Geometry check sheet. Reference: the model listing, model coordinates, mm. A direction names the side the tool comes from. Coordinates: 2 decimals unless noted, no trailing zeros. Loops run counter-clockwise (first coordinate to the right, second up) from the corner with the lowest first, then second, coordinate; pieces in that order, holes last.
from build123d import *

# Parameters (mm, degrees)
EXTRUSION1_DEPTH = 89
ESQUISSE2_R      = 1.5
ESQUISSE2_W      = 18.5
ESQUISSE2_H      = 20
ESQUISSE2_H_2    = 21.5
EXTRUSION2_DEPTH = 100
ESQUISSE3_R      = 1.5
EXTRUSION3_DEPTH = 100


with BuildPart() as part:
    # Esquisse1 → Extrusion1 (new body)
    with BuildSketch(Plane.XY):
        Polygon((-24.93137059, 6.591473684), (-24.93137059, -13.408526316), (-4.93137059, -13.408526316), (-4.93137059, -11.908526316), (-23.43137059, -11.908526316), (-23.43137059, 6.591473684), align=None)
    extrude(amount=EXTRUSION1_DEPTH)

    # Esquisse2 → Extrusion2 (cut)
    with BuildSketch(Plane(origin=(0, -11.908526316, 0), x_dir=(-1, 0, 0), z_dir=(0, 1, 0))):
        with Locations((14.93137059, 59)):
            Circle(ESQUISSE2_R)
        with Locations((14.93137059, 30)):
            Circle(ESQUISSE2_R)
        with Locations((14.18137059, 79)):
            Rectangle(ESQUISSE2_W, ESQUISSE2_H)
        with Locations((14.18137059, 10.75)):
            Rectangle(ESQUISSE2_W, ESQUISSE2_H_2)
    extrude(amount=-EXTRUSION2_DEPTH, mode=Mode.SUBTRACT)

    # Esquisse3 → Extrusion3 (cut)
    with BuildSketch(Plane(origin=(-23.43137059, 0, 0), x_dir=(0, 0, -1), z_dir=(1, 0, 0))):
        with Locations((-77.5, -3.408526316)):
            Circle(ESQUISSE3_R)
        with Locations((-10, -3.408526316)):
            Circle(ESQUISSE3_R)
    extrude(amount=-EXTRUSION3_DEPTH, mode=Mode.SUBTRACT)


solid = part.part
1) Material ranges on probe 1 along Y at (x, z) = (-23.9, 77.5); probe 2 along X at (y, z) = (4.25, 53.5); probe 3 along Y at (x, z) = (-21, 64.5), recorded low to high.
Data:
probe 1: y = -13.41 to -4.91, -1.91 to 6.59
probe 2: x = -24.93 to -23.43
probe 3: y = -13.41 to -11.91
2) Section check D-D on x = -22.25. Record the cut outline in (y, z), and give its area (4 significant figures).
Data:
outline: (-13.41, 21.5) - (-11.91, 21.5) - (-11.91, 69) - (-13.41, 69) - close
area: 71.25 mm2
3) Section check C-C on y = 1.75. Record the cut outline in (x, z).
Data:
outline: (-24.93, 0) - (-23.43, 0) - (-23.43, 89) - (-24.93, 89) - close
4) Depth check by flat-ended pin: pin 1 (8 mm diameter, centred on x = -14.5, z = 51, fed in from +Y); pin 2 (10 mm diameter, centred on y = -6, z = 48, fed in from +X); pin 3 (0.8 mm diameter, centred on x = -13, y = -12.5, fed in from -Z); pin 4 (1.8 mm diameter, centred on y = -3.41, z = 77.5, fed in from -X). Enter the tip coordinate at first touch or a pass-through.
Data:
pin 1: stops at y = -11.91
pin 2: stops at x = -23.43
pin 3: stops at z = 21.5
pin 4: passes through
5) Section check A-A on z = 77.5. Record the cut outline in (x, y).
Data:
outline: (-24.93, -13.41) - (-23.43, -13.41) - (-23.43, -4.91) - (-24.93, -4.91) - close; (-24.93, -1.91) - (-23.43, -1.91) - (-23.43, 6.59) - (-24.93, 6.59) - close
6) Access from +Z, -Z, +X, -X, +Y, -Y to the whole of each face (thin tool, end or side, straight path). Record for faces 4 (the flat face through (-14, -11.909, 45)), 5 (the flat face through (-14, -13, 69)), 6 (the flat face through (-14, -13, 21.5)).
Data:
face 4: +Z, -Z, +X, +Y
face 5: +Z, +X, +Y, -Y
face 6: -Z, +X, +Y, -Y
7) Mould release check, pull along Y, two halves, no side actions. Record for faces 1 (the flat face through (-15, -13.409, 44)), 2 (the cylindrical face through (-24.17, -2.96, 76.07)), 3 (the cylindrical face through (-14.736, -12.648, 60.487)): +Y half, -Y half, draft (parallel to the pull), parting line (faces both ways), or undercut.
Data:
face 1: -Y half
face 2: undercut
face 3: draft
8) Section check B-B on z = 68. Record the cut outline in (x, y).
Data:
outline: (-24.93, -13.41) - (-4.93, -13.41) - (-4.93, -11.91) - (-23.43, -11.91) - (-23.43, 6.59) - (-24.93, 6.59) - close
